Study the drawing (mm; zero at the part's minimum x, y, z) and answer. Give positions to 0.01 mm unless a question says otherwise; leave off trailing zeros. Write each loop counter-clockwise with the first axis right and the second up, starting at its lowest first coordinate (ties: lowest second). Pieces come first, ordered by that corner, then holes. Notation, with made-up numbers: (32, 63.25) - (64, 63.25) arc R14 cw to (64, 89.25) - close; hole circle Ø10 at (22.25, 53.25). An arc over 180 degrees is marked (long way). Write each question's results on one line, items separated by ' | '. Start each with the question number.
Q1. Find the intervals of material crossed by probe 1 along Y at (x, z) = (22.75, 14); probe 2 along Z at (x, y) = (2, 14) (1 decimal); probe 3 along X at (y, z) = (4.5, 15), in increasing order.
Q2. Flat-ended cylindrical pins translate along their axes: pin 1 Ø4 at (x, y) = (25.5, 22) entering from -Z (1 decimal); pin 2 Ø1 at (y, z) = (17, 6.5) entering from +X; pin 3 Ø1 at (y, z) = (20.5, 24.5) entering from -X; pin 4 Ø4.5 at (x, y) = (14.29, 12.7) entering from -Z. Find the tip coordinate at first contact, or state that the pin passes through.
Q3. Section A-A (y = 12.7) is taken. Determine the outline of the cut face in (x, z) (1 decimal), plus the area to 3 significant figures.
Q4. Section C-C (y = 19) is taken. Determine the outline of the cut face in (x, z) (1 decimal).
Q5. Section B-B (y = 4) is taken. Determine the outline of the cut face in (x, z) (1 decimal).
Q6. For a pull along X with two mould halves and no side action, classify the marked faces 1, 2, 3 and 4 as pulls with the +X half, pulls with the -X half, needs draft (parallel to the pull), parting line crosses it, or undercut.
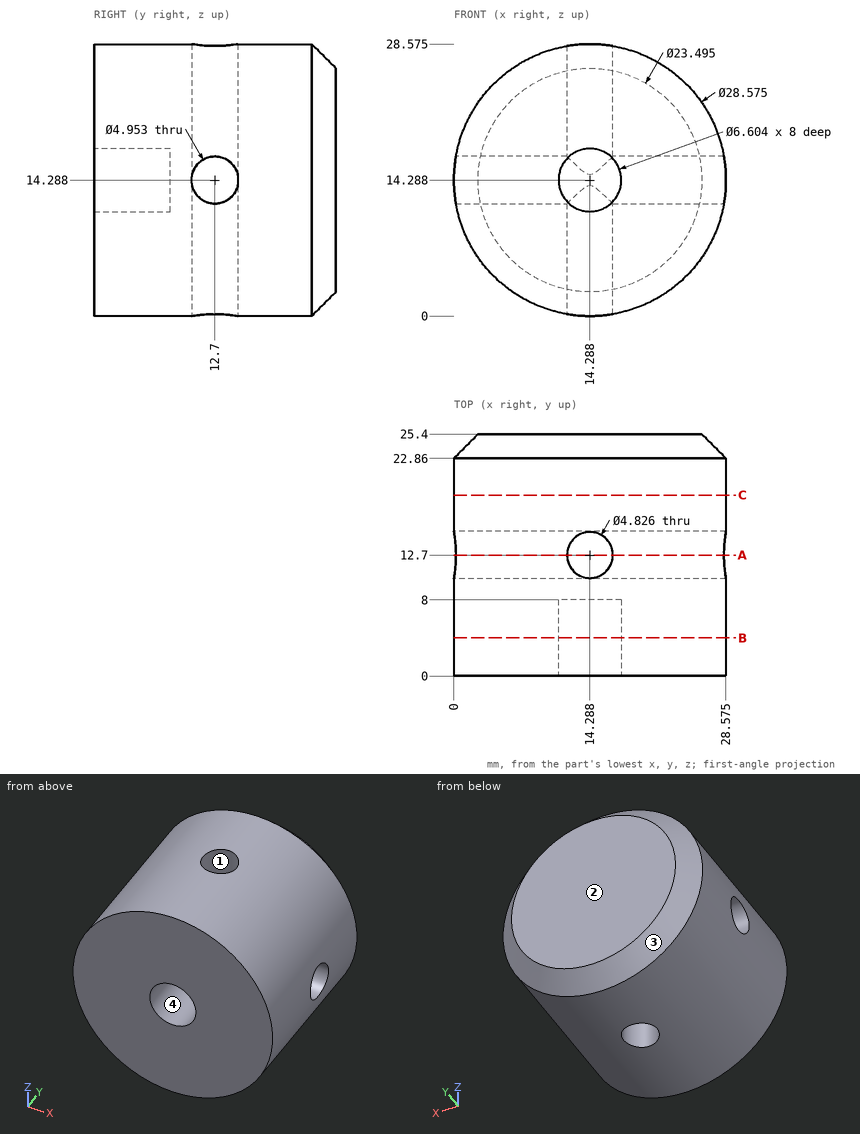
Answers below:
1) probe 1: y = 0 to 10.24, 15.16 to 25.4 | probe 2: z = 7 to 12.2, 16.4 to 21.6 | probe 3: x = 0.02 to 11.06, 17.51 to 28.56
2) pin 1: stops at z = 3.4 | pin 2: stops at x = 26.58 | pin 3: stops at x = 3.81 | pin 4: passes through
3) outline: (0.2, 11.8) arc R14.3 ccw to (11.9, 0.2) - (11.9, 11.8) - close; (0.2, 16.8) - (11.9, 16.8) - (11.9, 28.4) arc R14.3 ccw to start; (16.7, 0.2) arc R14.3 ccw to (28.4, 11.8) - (16.7, 11.8) - close; (16.7, 16.8) - (28.4, 16.8) arc R14.3 ccw to (16.7, 28.4) - close | area: 387 mm2
4) outline: circle Ø28.6 at (14.3, 14.3)
5) outline: circle Ø28.6 at (14.3, 14.3); hole circle Ø6.6 at (14.3, 14.3)
6) face 1: undercut | face 2: needs draft | face 3: parting line crosses it | face 4: undercut
